Read the model definition and answer for the solid it produces. Units are mm, in the model's axes. Face numbers are marked on the shaded views. A direction names the side the tool comes from. Give positions to 0.01 mm unless a question says otherwise; leave off trailing zeros. Order: outer loops, then holes, each group sorted by start corner. A loop starts at its lowest first (then second) coordinate and runs counter-clockwise, first axis right, second up.
Item 1: Which of the six approach directions +Z, -Z, +X, -X, +Y, -Y give full straight-line access (tool end or side, diameter ignored) to the marked faces 1, 2 and 3?
Item 2: A cutting plane is placed at C-C (y = 20). Write down the section's boundary in (x, z), plus the area to 3 significant figures.
Item 3: Given pin 1 Ø5 at (x, z) = (-11, -33.5) entering from +Y; pin 2 Ø4 at (y, z) = (25.5, -31.5) entering from +X; pin 3 Ø1.6 at (x, z) = (-52.5, -20.5) entering from -Y; pin 4 Ø17.5 at (x, y) = (-52.5, 14.5) entering from +Z, each flat-ended and moving along its own axis, determine where each tip first touches the part or whether it passes through.
Item 4: A cutting plane is placed at B-B (z = -18). Write down the section's boundary in (x, y).
Item 5: Find the intervals of material crossed by line 1 along Z through (x, y) = (-16.5, 8.5); line 2 along Z through (x, y) = (-9, 1); line 3 along Z through (x, y) = (-34, 19.5), in increasing order.
Item 6: The mould has two halves that part along Z. Classify the marked faces 4, 5, 6 and 7: +Z half, -Z half, draft (parallel to the pull), parting line (faces both ways), or undercut.
Item 7: A cutting plane is placed at A-A (x = -9.55). Write down the section's boundary in (y, z).
Item 8: A cutting plane is placed at D-D (x = -36.5). Write down the section's boundary in (y, z), plus the area to 4 significant figures.
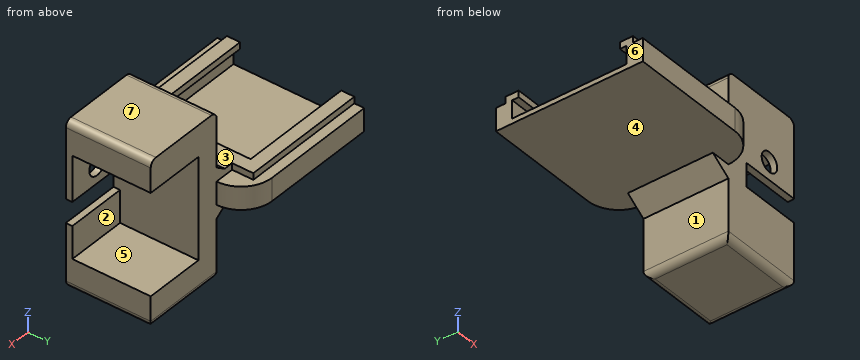
Autodesk Inventor part; units mm, degrees
ref_plane "YZ Plane" through (0, 0, 0) normal (1, 0, 0) x (0, 1, 0)
ref_plane "XZ Plane" through (0, 0, 0) normal (0, 1, 0) x (-1, 0, 0)
ref_plane "XY Plane" through (0, 0, 0) normal (0, 0, 1) x (1, 0, 0)
sketch "Sketch1" plane through (0, 0, 0) normal (0, 1, 0) x (-1, 0, 0)
  line L0 (0, 0) -> (25.4, 0)
  line L1 (25.4, 0) -> (25.4, -50)
  line L2 (25.4, -50) -> (0, -50)
  line L3 (0, -50) -> (0, 0)
  dimension "d0" = 25.4
  dimension "d1" = 50
extrude "Extrusion1" add sketch "Sketch1" along normal blind 5
sketch "Sketch2" plane through (0, 5, 0) normal (0, 1, 0) x (1, 0, 0)
  line L0 (-25.4, 0) -> (0, 0)
  line L1 (-25.4, 0) -> (0, 0)
  line L2 (0, 0) -> (0, 9.5)
  line L3 (0, 9.5) -> (-25.4, 9.5)
  line L4 (-25.4, 9.5) -> (-25.4, 0)
  line L5 (0, 0) -> (0, 50) construction
  line L6 (-25.4, 50) -> (-25.4, 0) construction
  line L7 (0, 50) -> (-25.4, 50)
  line L8 (-25.4, 50) -> (-25.4, 40.5)
  line L9 (-25.4, 40.5) -> (0, 40.5)
  line L10 (0, 40.5) -> (0, 50)
  line L11 (-18.4, 4) -> (-3.2, 4) construction
  line L12 (-3.2, 4) -> (-3.2, 46) construction
  line L13 (-3.2, 46) -> (-18.4, 46) construction
  line L14 (-18.4, 46) -> (-18.4, 4) construction
  line L15 (-10.8, 6.25) -> (-10.8, 43.75) construction
  line L16 (-3.2, 9.5) -> (-18.4, 9.5) construction
  line L17 (-18.4, 40.5) -> (-3.2, 40.5) construction
  line L18 (-12.3588, 9.5) -> (-12.3588, 40.5) construction
  line L19 (-25.4, 40.5) -> (-18.4, 40.5)
  line L20 (-18.4, 40.5) -> (-18.4, 9.5)
  line L21 (-18.4, 9.5) -> (-25.4, 9.5)
  line L22 (-25.4, 9.5) -> (-25.4, 40.5)
  point P0 (-10.8, 25)
  point P1 (-18.4, 25)
  point P2 (-10.8, 4)
  point P3 (-12.3588, 25)
  dimension "d4" = 42
  dimension "d5" = 15.2
  dimension "d6" = 37.5
  dimension "d7" = 31
  dimension "d14" = 7
extrude "Extrusion2" add sketch "Sketch2" along normal blind 21
sketch "Sketch6" plane through (0, 0, 0) normal (0, -1, 0) x (1, 0, 0)
  circle A0 centre (-9.55, -18) radius 3
  line L0 (0, -50) -> (0, 0)
  line L1 (0, 0) -> (-25.4, 0)
  dimension "d24" = 6
  dimension "d25" = 9.55
  dimension "d26" = 18
extrude "Extrusion6" cut sketch "Sketch6" against normal up to next
fillet "Fillet1" radius 2 6 edges at (-25.4, 13, 0) (0, 13, 0) (-25.4, 13, -50) (-12.7, 0, -50) (-12.7, 26, -50) (0, 13, -50)
sketch "Sketch8" plane through (-25.4, 0, -48) normal (-1, 0, 0) x (0, 0, 1)
  line L0 (38.5, 26) -> (7.5, 26)
  line L1 (46, 0) -> (0, 0)
  line L2 (23, 13) -> (23, 35.5)
  line L3 (23, 13) -> (23, -9.5)
  line L4 (23, 35.5) -> (27, 35.5)
  line L5 (23, -9.5) -> (20, -9.5)
  line L6 (20, -9.5) -> (27, -9.5)
  line L7 (27, -9.5) -> (27, 35.5)
  line L8 (27, 35.5) -> (20, 35.5)
  line L9 (20, 35.5) -> (20, -9.5)
  point P0 (48, 0)
  point P1 (23, -9.5)
  point P2 (23, 35.5)
  dimension "d33" = 22.5
  dimension "d34" = 22.5
  dimension "d35" = 4
  dimension "d36" = 3
extrude "Extrusion8" add sketch "Sketch8" along normal blind 45
sketch "Sketch9" plane through (-70.4, 0, -48) normal (-1, 0, 0) x (0, 0, 1)
  line L0 (27, -9.5) -> (27, 35.5)
  line L1 (20, 35.5) -> (20, -9.5)
  line L2 (23.5, 13) -> (23.5, -4.5)
  line L3 (23.5, -4.5) -> (27, -4.5)
  line L4 (23.5, 13) -> (23.5, 30.5)
  line L5 (23.5, 30.5) -> (27, 30.5)
  line L6 (27, 30.5) -> (27, -4.5)
  point P0 (48, 0)
  dimension "d39" = 17.5
  dimension "d40" = 17.5
extrude "Extrusion9" cut sketch "Sketch9" against normal blind 37
sketch "Sketch10" plane through (-70.4, -4.5, -24.5) normal (0, 0, 1) x (1, 0, 0)
  line L0 (0, 0) -> (0, 35)
  line L1 (37, 35) -> (37, 0)
  line L2 (0, 0) -> (37, 0)
  line L3 (37, 0) -> (37, 35)
  line L4 (37, 35) -> (0, 35)
  line L5 (0, 35) -> (0, 0)
  point P0 (70.4, 4.5)
extrude "Extrusion10" cut sketch "Sketch10" against normal blind 2
sketch "Sketch11" plane through (-25.4, -9.5, -21) normal (0, 0, 1) x (1, 0, 0)
  line L0 (-8, 5) -> (-45, 5)
  line L1 (-45, 5) -> (-45, 3)
  line L2 (-45, 0) -> (-45, 5)
  line L3 (-6, 5) -> (-6, 3)
  line L4 (-6, 3) -> (-45, 3)
  line L5 (-8, 40) -> (-8, 5)
  line L6 (-6, 5) -> (-6, 42)
  line L7 (-6, 42) -> (-45, 42)
  line L8 (-45, 45) -> (-45, 0)
  line L9 (-45, 40) -> (-8, 40)
  line L10 (-45, 42) -> (-45, 40)
  line L11 (-45, 40) -> (-45, 38)
  line L12 (-45, 38) -> (-10, 38)
  line L13 (-10, 38) -> (-10, 7)
  line L14 (-10, 7) -> (-45, 7)
  line L15 (-45, 5) -> (-45, 7)
  point P0 (25.4, 9.5)
  dimension "d45" = 2
  dimension "d46" = 2
  dimension "d48" = 2
  dimension "d49" = 35
  dimension "d50" = 31
extrude "Extrusion11" add sketch "Sketch11" along normal blind 2 contours L5 L9 L8 L7 L6 L3 L4 L1 L0 | L0 L8 L14 L13 L12 L9 L5
sketch "Sketch12" plane through (0, 5, 0) normal (0, 1, 0) x (1, 0, 0)
  line L0 (-18.4, 40.5) -> (-18.4, 9.5)
  line L1 (0, 40.5) -> (-18.4, 40.5)
  line L2 (-18.4, 9.5) -> (0, 9.5)
  line L3 (0, 9.5) -> (0, 40.5)
  line L4 (0, 40.5) -> (-18.4, 40.5)
  line L5 (-18.4, 40.5) -> (-18.4, 9.5)
  circle A0 centre (-9.55, 18) radius 3
  circle A1 centre (-9.55, 18) radius 3
  point P0 (0, 0)
extrude "Extrusion12" cut sketch "Sketch12" against normal blind 3
fillet "Fillet2" radius 9.5 2 edges at (-25.4, 35.5, -24.5) (-25.4, -9.5, -24.5)
sketch "Sketch13" plane through (0, 0, 0) normal (0, -1, 0) x (1, 0, 0)
  line L0 (-31.4, -21) -> (-31.4, -19)
  line L1 (-28.5437, -19) -> (-25.4, -16.7988)
  line L2 (-25.4, -2) -> (-25.4, -21)
  line L3 (-31.4, -21) -> (-24.0754, -21) construction
  line L4 (-25.4, -16.7988) -> (-25.4, -21)
  line L5 (-25.4, -21) -> (-31.4, -21)
  line L6 (-31.4, -19) -> (-70.4, -19)
  line L7 (-31.4, -19) -> (-28.5437, -19)
  line L8 (-25.4, -28) -> (-34.9, -28)
  line L9 (-31.4, -28) -> (-25.4, -32.2012)
  line L10 (-25.4, -28) -> (-25.4, -48)
  line L11 (-31.4, -28) -> (-24.0754, -28) construction
  line L12 (-25.4, -32.2012) -> (-25.4, -28)
  line L13 (-25.4, -28) -> (-31.4, -28)
  point P0 (0, 0)
  dimension "d56" = 35
  dimension "d57" = 35
extrude "Extrusion13" add sketch "Sketch13" against normal up to surface (26 mm away)
sketch "Sketch14" plane through (0, 2, 0) normal (0, 1, 0) x (1, 0, 0)
  line L0 (-18.4, 9.5) -> (-18.4, 40.5)
  line L1 (0, 40.5) -> (0, 9.5)
  line L2 (-18.4, 23.418) -> (0, 23.418)
  line L3 (0, 23.418) -> (0, 30.6155)
  line L4 (0, 30.6155) -> (-18.4, 30.6155)
  line L5 (-18.4, 30.6155) -> (-18.4, 23.418)
  point P0 (0, 0)
  point P1 (0, 23.418)
extrude "Extrusion14" cut sketch "Sketch14" against normal through all
properties part number "Tilt_Camera_Servo_Mount"
Response values:
1. face 1: -Z, -X, +Y, -Y
1. face 2: +X, +Y
1. face 3: +Z, -X, +Y, -Y
2. outline: (-70.4, -28) - (-31.4, -28) - (-25.4, -32.2) - (-25.4, -48) arc R2 ccw to (-23.4, -50) - (-2, -50) arc R2 ccw to (0, -48) - (0, -40.5) - (-18.4, -40.5) - (-18.4, -9.5) - (0, -9.5) - (0, -2) arc R2 ccw to (-2, 0) - (-23.4, 0) arc R2 ccw to (-25.4, -2) - (-25.4, -16.8) - (-28.54, -19) - (-35.4, -19) - (-35.4, -21) - (-33.4, -21) - (-33.4, -26.5) - (-70.4, -26.5) - close
2. area: 844 mm2
3. pin 1: stops at y = 2
3. pin 2: stops at x = -18.4
3. pin 3: stops at y = -9.5
3. pin 4: stops at z = -26.5
4. outline: (-27.12, 0) - (-12.55, 0) - (-12.55, 2) - (-18.4, 2) - (-18.4, 26) - (-27.12, 26) - close; (-6.55, 0) - (0, 0) - (0, 2) - (-6.55, 2) - close
5. line 1: z = -50 to -40.5, -9.5 to 0
5. line 2: z = -49.73 to -30.62, -23.42 to -20.95, -15.05 to 0
5. line 3: z = -28 to -26.5, -21 to -19
6. face 4: -Z half
6. face 5: undercut
6. face 6: draft
6. face 7: +Z half
7. outline: (0, -48) arc R2 ccw to (2, -50) - (24, -50) arc R2 ccw to (26, -48) - (26, -40.5) - (2, -40.5) - (2, -30.62) - (0, -30.62) - close; (0, -23.42) - (2, -23.42) - (2, -21) - (0, -21) - close; (0, -15) - (2, -15) - (2, -9.5) - (26, -9.5) - (26, 0) - (0, 0) - close
8. outline: (-9.5, -28) - (35.5, -28) - (35.5, -21) - (32.5, -21) - (32.5, -19) - (28.5, -19) - (28.5, -21) - (30.5, -21) - (30.5, -26.5) - (-4.5, -26.5) - (-4.5, -21) - (-2.5, -21) - (-2.5, -19) - (-6.5, -19) - (-6.5, -21) - (-9.5, -21) - close
8. area: 138.5 mm2
